from build123d import *
from build123d.topology import SkipClean

# Parameters (mm, degrees)
SKETCH1_R                                        = 40
BOSS_EXTRUDE1_DEPTH                              = 10.75
CUT_EXTRUDE1_DEPTH                               = 6
CUT_EXTRUDE2_DEPTH                               = 6
SKETCH4_W                                        = 6
SKETCH4_H                                        = 5.601183879
CUT_EXTRUDE3_DEPTH                               = 0.706099456
SKETCH5_W                                        = 5.601183879
SKETCH5_H                                        = 6
CUT_EXTRUDE4_DEPTH                               = 4.589754851
SKETCH6_W                                        = 7
SKETCH6_H                                        = 6
CUT_EXTRUDE5_DEPTH                               = 7.355277629
CUT_EXTRUDE6_REACH                               = 59.241
SKETCH8_W                                        = 12.651131937
SKETCH8_H                                        = 7
CUT_EXTRUDE7_DEPTH                               = 6
BOSS_EXTRUDE2_START                              = 8.75
BOSS_EXTRUDE2_DEPTH                              = 8.75
SKETCH10_W                                       = 12.651131937
SKETCH10_H                                       = 7
CUT_EXTRUDE8_DEPTH                               = 6
SKETCH11_W                                       = 12.651131937
SKETCH11_H                                       = 7
CUT_EXTRUDE9_DEPTH                               = 6
SKETCH12_W                                       = 13
SKETCH12_H                                       = 2
BOSS_EXTRUDE3_DEPTH                              = 4
DRAFT1_ANGLE                                     = 68.007906367
DRAFT2_ANGLE                                     = 21.992093633
M4_CLEARANCE_HOLE1_D                             = 4.66
CBORE_FOR_M4_HEX_HEAD_MACHINE_SCREW1_AT_COUNT    = 2
CBORE_FOR_M4_HEX_HEAD_MACHINE_SCREW1_AT_PITCH    = 43.22206146
CBORE_FOR_M4_HEX_HEAD_MACHINE_SCREW1_2_COUNT     = 2
CBORE_FOR_M4_HEX_HEAD_MACHINE_SCREW1_2_PITCH     = 71
CBORE_FOR_M4_HEX_HEAD_MACHINE_SCREW1_3_COUNT     = 2
CBORE_FOR_M4_HEX_HEAD_MACHINE_SCREW1_3_PITCH     = 56.328087161
F_8_8_8_8_DIAMETER_HOLE1_D                       = 8.8
F_8_8_8_8_DIAMETER_HOLE1_DEPTH                   = 10.75
CBORE_FOR_M4_HEX_HEAD_MACHINE_SCREW2_D           = 4.35
CBORE_FOR_M4_HEX_HEAD_MACHINE_SCREW2_CBORE_D     = 7.8
CBORE_FOR_M4_HEX_HEAD_MACHINE_SCREW2_CBORE_DEPTH = 8
CHAMFER1_SIZE                                    = 2
CHAMFER2_SIZE                                    = 1.5311569
CHAMFER2_SIZE2                                   = 1.474148544
FILLET1_R                                        = 0.5


with BuildPart() as part:
    # Sketch1 → Boss-Extrude1 (new body)
    with BuildSketch(Plane(origin=(0, 10.75, 0), x_dir=(1, 0, 0), z_dir=(0, 1, 0))):
        with Locations(Location((0, 0, 0), (0, 0, 90))):
            Circle(SKETCH1_R)
        Polygon((-13.295854308, -23.598274832), (-13.295854308, -17.3), (-12.589754851, -15.901183879), (5.76268576, -15.901183879), align=None, mode=Mode.SUBTRACT)
    extrude(amount=-BOSS_EXTRUDE1_DEPTH)

    # Sketch2 → Cut-Extrude1 (cut)
    with BuildSketch(Plane(origin=(0, 10.75, 0), x_dir=(-1, 0, 0), z_dir=(0, 1, 0))):
        Polygon((12.589754851, 15.901183879), (13.295854308, 15.901183879), (13.295854308, 17.3), align=None)
    extrude(amount=-CUT_EXTRUDE1_DEPTH, mode=Mode.SUBTRACT)

    # Sketch3 → Cut-Extrude2 (cut)
    with BuildSketch(Plane(origin=(0, 10.75, 0), x_dir=(-1, 0, 0), z_dir=(0, 1, 0))):
        with BuildLine():
            Line((38.651131937, 10.3), (-38.651131937, 10.3))
            ThreePointArc((-38.651131937, 10.3), (0, -40), (38.651131937, 10.3))
        make_face()
    extrude(amount=-CUT_EXTRUDE2_DEPTH, mode=Mode.SUBTRACT)

    # Sketch4 → Cut-Extrude3 (cut)
    with BuildSketch(Plane(origin=(-13.295854308, 0, 0), x_dir=(0, -1, 0), z_dir=(-1, 0, 0))):
        with Locations((-7.75, 13.10059194)):
            Rectangle(SKETCH4_W, SKETCH4_H)
    extrude(amount=-CUT_EXTRUDE3_DEPTH, mode=Mode.SUBTRACT)

    # Sketch5 → Cut-Extrude4 (cut)
    with BuildSketch(Plane.ZY.offset(12.589754851)):
        with Locations((13.10059194, 7.75)):
            Rectangle(SKETCH5_W, SKETCH5_H)
    extrude(amount=-CUT_EXTRUDE4_DEPTH, mode=Mode.SUBTRACT)

    # Sketch6 → Cut-Extrude5 (cut)
    with BuildSketch(Plane(origin=(-13.295854308, 0, 0), x_dir=(0, 0, -1), z_dir=(1, 0, 0))):
        with Locations((-13.8, 7.75)):
            Rectangle(SKETCH6_W, SKETCH6_H)
    extrude(amount=-CUT_EXTRUDE5_DEPTH, mode=Mode.SUBTRACT)

    # Sketch7 → Cut-Extrude6 (cut, up to next)
    with BuildSketch(Plane.XZ.offset(-2), mode=Mode.PRIVATE) as cut_extrude6_sk1:
        with BuildLine():
            Line((38.651131937, 10.3), (-38.651131937, 10.3))
            ThreePointArc((-38.651131937, 10.3), (0, -40), (38.651131937, 10.3))
        make_face()
    cut_extrude6_tool1 = extrude(cut_extrude6_sk1.sketch, amount=-CUT_EXTRUDE6_REACH, mode=Mode.PRIVATE) & part.part
    add(cut_extrude6_tool1.solids().sort_by_distance((0, 2, -11.566508))[0], mode=Mode.SUBTRACT)

    # Sketch8 → Cut-Extrude7 (cut)
    with BuildSketch(Plane(origin=(0, 10.75, 0), x_dir=(-1, 0, 0), z_dir=(0, 1, 0))):
        with Locations((-14.325565969, 13.8)):
            Rectangle(SKETCH8_W, SKETCH8_H)
    extrude(amount=-CUT_EXTRUDE7_DEPTH, mode=Mode.SUBTRACT)

    # Sketch9 → Boss-Extrude2 (add)
    with SkipClean():  # the faces are left unmerged after this step: merging them gives an invalid solid
        with BuildSketch(Plane(origin=(0, 2, 0), x_dir=(-1, 0, 0), z_dir=(0, 1, 0)).offset(BOSS_EXTRUDE2_START)):
            with BuildLine():
                Line((-38.651131937, -10.3), (38.651131937, -10.3))
                ThreePointArc((38.651131937, -10.3), (0, -40), (-38.651131937, -10.3))
            make_face()
        extrude(amount=-BOSS_EXTRUDE2_DEPTH)
    add(part.part.scale(1), mode=Mode.REPLACE)  # the faces are merged on a copy

    # Sketch10 → Cut-Extrude8 (cut)
    with BuildSketch(Plane(origin=(0, 10.75, 0), x_dir=(-1, 0, 0), z_dir=(0, 1, 0))):
        with Locations((-14.325565969, -13.8)):
            Rectangle(SKETCH10_W, SKETCH10_H)
    extrude(amount=-CUT_EXTRUDE8_DEPTH, mode=Mode.SUBTRACT)

    # Sketch11 → Cut-Extrude9 (cut)
    with BuildSketch(Plane(origin=(0, 10.75, 0), x_dir=(-1, 0, 0), z_dir=(0, 1, 0))):
        with Locations((14.325565969, -13.8)):
            Rectangle(SKETCH11_W, SKETCH11_H)
    extrude(amount=-CUT_EXTRUDE9_DEPTH, mode=Mode.SUBTRACT)

    # Sketch12 → Boss-Extrude3 (add)
    with BuildSketch(Plane(origin=(0, 2, 0), x_dir=(-1, 0, 0), z_dir=(0, 1, 0))):
        Rectangle(SKETCH12_W, SKETCH12_H)
    extrude(amount=BOSS_EXTRUDE3_DEPTH)

    # Draft1
    draft1_faces = [part.faces().sort_by_distance(p)[0] for p in [
        (-2.297176197, 4.989704408, 15.901183879),
    ]]
    draft(draft1_faces, Plane(origin=(-8, 0, 0), x_dir=(0, 0, -1), z_dir=(-1, 0, 0)), DRAFT1_ANGLE)

    # Draft2
    draft2_faces = [part.faces().sort_by_distance(p)[0] for p in [
        (-13.295854308, 5.375, 20.449137416),
    ]]
    draft(draft2_faces, Plane(origin=(-20.651131937, 10.75, 17.3), x_dir=(-1, 0, 0), z_dir=(0, 0, -1)), DRAFT2_ANGLE)

    # M4 Clearance Hole1 (through all)
    with Locations(Plane(origin=(0, 0, 0), x_dir=(-1, 0, 0), z_dir=(0, -1, 0))):
        with Locations((-4.307478356, -12.879228634), (4.307478356, 12.879228634), (-4.307478356, 12.879228634), (4.307478356, -12.879228634)):
            Hole(M4_CLEARANCE_HOLE1_D / 2)

    # Sketch15 → CBORE for M4 Hex Head Machine Screw1 (revolve, cut)
    with BuildSketch(Plane(origin=(25.102290732, 10.75, -25.102290732), x_dir=(0, 0, 1), z_dir=(1, 0, 0))):
        Polygon((0, 0), (0, 10.75), (2.4, 10.75), (2.4, 5), (4, 5), (4, 1.32), (5.32, 0), align=None)
    cbore_for_m4_hex_head_machine_screw1 = revolve(axis=Axis((25.102290732, 17.1, -25.102290732), (0, -1, 0)), mode=Mode.SUBTRACT)

    # CBORE for M4 Hex Head Machine Screw1 at: CBORE for M4 Hex Head Machine Screw1 ×2
    with Locations(*[Vector(-0.9914448613738109, 0, -0.13052619222004783) * (i * CBORE_FOR_M4_HEX_HEAD_MACHINE_SCREW1_AT_PITCH) for i in range(1, CBORE_FOR_M4_HEX_HEAD_MACHINE_SCREW1_AT_COUNT)]):
        add(cbore_for_m4_hex_head_machine_screw1, mode=Mode.SUBTRACT)

    # CBORE for M4 Hex Head Machine Screw1 2: CBORE for M4 Hex Head Machine Screw1 ×2
    with Locations(*[Vector(-0.7071067811865434, 0, 0.7071067811865517) * (i * CBORE_FOR_M4_HEX_HEAD_MACHINE_SCREW1_2_PITCH) for i in range(1, CBORE_FOR_M4_HEX_HEAD_MACHINE_SCREW1_2_COUNT)]):
        add(cbore_for_m4_hex_head_machine_screw1, mode=Mode.SUBTRACT)

    # CBORE for M4 Hex Head Machine Screw1 3: CBORE for M4 Hex Head Machine Screw1 ×2
    with Locations(*[Vector(-0.13052619222004894, 0, 0.9914448613738108) * (i * CBORE_FOR_M4_HEX_HEAD_MACHINE_SCREW1_3_PITCH) for i in range(1, CBORE_FOR_M4_HEX_HEAD_MACHINE_SCREW1_3_COUNT)]):
        add(cbore_for_m4_hex_head_machine_screw1, mode=Mode.SUBTRACT)

    # Ø8.8 (8.8) Diameter Hole1
    with Locations(Plane(origin=(0, 0, 0), x_dir=(-1, 0, 0), z_dir=(0, -1, 0))):
        with Locations((33, 0), (-33, 0)):
            Hole(F_8_8_8_8_DIAMETER_HOLE1_D / 2, depth=F_8_8_8_8_DIAMETER_HOLE1_DEPTH)

    # CBORE for M4 Hex Head Machine Screw2 (through all)
    with Locations(Plane(origin=(0, 0, 0), x_dir=(-1, 0, 0), z_dir=(0, -1, 0))):
        with Locations((31.185228347, -15.889667491), (0, -35), (-31.185228347, -15.889667491), (31.185228347, 15.889667491), (0, 35), (-31.185228347, 15.889667491)):
            CounterBoreHole(CBORE_FOR_M4_HEX_HEAD_MACHINE_SCREW2_D / 2, CBORE_FOR_M4_HEX_HEAD_MACHINE_SCREW2_CBORE_D / 2, CBORE_FOR_M4_HEX_HEAD_MACHINE_SCREW2_CBORE_DEPTH)

    # Chamfer1
    # the kernel refuses this chamfer: 2 mm, written as the material it takes off along each edge
    with BuildSketch(Plane(origin=(8, 4.75, -10.3), x_dir=(0, -0.9996219169112968, 0.027495876610586473), z_dir=(1, 0, 0)), Plane(origin=(-20.651131937, 4.75, -10.3), x_dir=(0, -0.9996219169112968, 0.027495876610586473), z_dir=(1, 0, 0)), Plane(origin=(-8, 4.75, 10.3), x_dir=(0, -0.9996219169112968, -0.027495876610586462), z_dir=(-1, 0, 0)), Plane(origin=(20.651131937, 4.75, 10.3), x_dir=(0, -0.9996219169112968, -0.027495876610586473), z_dir=(-1, 0, 0))) as chamfer1_piece_1:
        Polygon((CHAMFER1_SIZE * 0.999621916911, CHAMFER1_SIZE * 0.0274958766106), (-CHAMFER1_SIZE * 0.0274958766106, CHAMFER1_SIZE * 0.999621916911), (0, 0), align=None)
    extrude(amount=12.651131937, mode=Mode.SUBTRACT)

    # Chamfer2
    chamfer2_edges = [part.edges().sort_by_distance(p)[0] for p in [
        (-10.04, 1.65, 10.85),
    ]]
    chamfer2_side = [part.faces().sort_by_distance(p)[0] for p in [
        (-11.717101205, 2.307785852, 14.1724161),
    ]]
    chamfer(chamfer2_edges, length=CHAMFER2_SIZE, length2=CHAMFER2_SIZE2, reference=chamfer2_side[0])

    # Fillet1
    fillet1_edges = [part.edges().sort_by_distance(p)[0] for p in [
        (0, 0, 40),
    ]]
    fillet(fillet1_edges, radius=FILLET1_R)


solid = part.part
Design review of the part built by this model. Coordinates are the model's own, in mm. A direction names the side the tool comes from. Give positions to 0.01 mm unless a question says otherwise; leave off trailing zeros. Answer as a JSON object with one key per item and string values.
Item 1: We need section A-A (z = -2). Count the separate pieces of the cut face and the enclosed holes in it, and give its area (3 significant figures).
Output values:
{"separate pieces": "3", "enclosed holes": "0", "area": "128 mm2"}
Item 2: Mouldability with a two-part tool opening along X and no side actions: class faces 5 (the face through (-2, 8, 37)), 6 (the face through (0, 4, -1)) as pulls with the +X half, pulls with the -X half, needs draft (parallel to the pull), parting line crosses it, or undercut.
Output values:
{"face 5": "undercut", "face 6": "needs draft"}
Item 3: Machinability: for faces 1 (the face through (-12.03, 2.41, 14.79)), 2 (the face through (-26, 8, 29)), 3 (the face through (-30.678, 3.944, 12.023)), 4 (the face through (-1, 6, 10.3)), which of the approach directions +Z, -Z, +X, -X, +Y, -Y give a long, thin tool a straight path to every point of the face, cutting with its end or side? Answer none if there is none.
Output values:
{"face 1": "+Y, -Y", "face 2": "+Y", "face 3": "-Y", "face 4": "+X, -X, +Y"}
Item 4: Wall thickness on line 1 along Z through (x, y) = (0, 4.25); line 2 along Z through (x, y) = (27, 3.25); line 3 along Z through (x, y) = (23, 3.5): over which ranges is each line inside the solid? List them lowest first.
Output values:
{"line 1": "z = -40 to -38.9, -31.1 to -10.3, -1 to 1, 10.3 to 31.1, 38.9 to 40", "line 2": "z = -29.51 to -26.57, -23.63 to -10.3, 10.3 to 29.51", "line 3": "z = -32.73 to -26.26, -23.94 to -10.3, 10.3 to 32.73"}
Item 5: For P1, Ø2.5, axis at x = 32.5, z = 17, coming from the -Y side; P2, Ø7.5, axis at x = 25.1, z = -25.1, coming from the +Y side; P3, Ø6, axis at x = 5.5, y = 1.5, coming from the +Z side, all flat-tipped, find the tip position at first contact; note any pin that passes through.
Output values:
{"P1": "stops at y = 8", "P2": "stops at y = 5.75", "P3": "stops at z = 39.92"}
